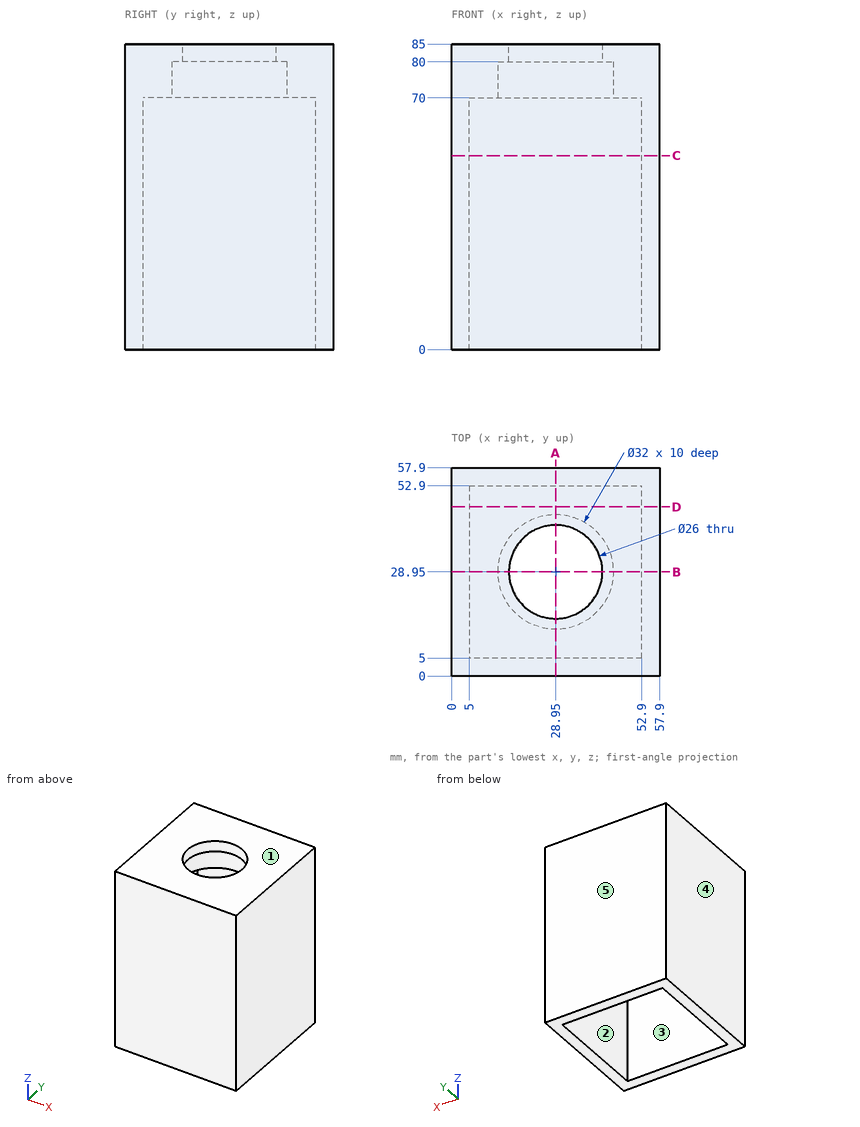
Geometry check sheet. Reference: drawing and pictorial views, mm from the part's lowest x, y, z. A direction names the side the tool comes from. Give positions to 0.01 mm unless a question says otherwise; leave off trailing zeros. Write each loop counter-clockwise with the first axis right and the second up, starting at its lowest first coordinate (ties: lowest second). Pieces come first, ordered by that corner, then holes. Notation, with made-up numbers: (-30.75, -32) - (24.25, -32) arc R24 cw to (24.25, 7) - close; hole circle Ø6 at (74.5, -34). An arc over 180 degrees is marked (long way). Use a Markdown table: item, result.
Q1. Set-up check for the marked faces 1 and 2: record each of +Z, -Z, +X, -X, +Y, -Y from which the full face is reachable in a straight line by a thin tool's end or side.
Computed:
| item | result |
|---|---|
| face 1 | +Z, +X, -X, +Y, -Y |
| face 2 | -Z |
Q2. Section check D-D, the plane y = 47. Enter the section's corners in (x, z).
Computed:
| item | result |
|---|---|
| outline | (0, 0) - (5, 0) - (5, 70) - (52.9, 70) - (52.9, 0) - (57.9, 0) - (57.9, 85) - (0, 85) - close |
Q3. Section check A-A, the plane x = 28.95. Enter the section's corners in (y, z).
Computed:
| item | result |
|---|---|
| outline | (0, 0) - (5, 0) - (5, 70) - (12.95, 70) - (12.95, 80) - (15.95, 80) - (15.95, 85) - (0, 85) - close; (41.95, 80) - (44.95, 80) - (44.95, 70) - (52.9, 70) - (52.9, 0) - (57.9, 0) - (57.9, 85) - (41.95, 85) - close |
Q4. Go/stop test with flat-tipped pins: P1, Ø6, axis at x = 14, y = 13.5, coming from the -Z side; P2, Ø14.5, axis at x = 27.5, y = 21, coming from the -Z side. Record where each tip stops, or that it passes through.
Computed:
| item | result |
|---|---|
| P1 | stops at z = 70 |
| P2 | stops at z = 80 |
Q5. Section check C-C, the plane z = 54. Enter the section's corners in (x, y), then the cut area to 3 significant figures.
Computed:
| item | result |
|---|---|
| outline | (0, 0) - (57.9, 0) - (57.9, 57.9) - (0, 57.9) - close; hole (5, 5) - (52.9, 5) - (52.9, 52.9) - (5, 52.9) - close |
| area | 1,060 mm² |
Q6. Draft check along Y on the marked faces 3, 4 and 5. Enter one of: pulls with the +Y half, pulls with the -Y half, needs draft (parallel to the pull), parting line crosses it, or undercut.
Computed:
| item | result |
|---|---|
| face 3 | undercut |
| face 4 | needs draft |
| face 5 | pulls with the +Y half |
Q7. Thickness scan on L1, parallel to X at y = 50.5, z = 50; L2, parallel to Y at x = 28.95, z = 73.75. Record the ranges inside material, lowest first. Write a range as [from, to].
Computed:
| item | result |
|---|---|
| L1 | x = [0, 5], [52.9, 57.9] |
| L2 | y = [0, 12.95], [44.95, 57.9] |
